Build history of the part. All positions in model axes, mm. A direction names the side the tool comes from. Give positions to 0.01 mm unless a question says otherwise; leave off trailing zeros. Loops run counter-clockwise (first coordinate to the right, second up) from the corner with the lowest first, then second, coordinate; pieces in that order, holes last.
1) Flat gauge pins, fed straight in: P1, Ø2.5, axis at y = 100, z = 2.5, coming from the +X side; P2, Ø3, axis at x = 21, z = 3, coming from the +Y side; P3, Ø1.5, axis at y = -6, z = 2.5, coming from the +X side. Where does each tip first touch, or does it go through?
2) Wall check: line 1 (X direction, y = 82, z = 1.9); line 2 (X direction, y = -49, z = 2.5); line 3 (X direction, y = -6, z = 1.35). Give the ranges that are in metal, low to high.
3) Band-saw the part on A-A on y = -64. List the corners of the cut face in (x, z).
4) Two-plate mould, pull along X, no slides. Class faces 4 (the flat face through (114.786, 13, 2)), 5 (the flat face through (120, -28.788, 2)), 6 (the flat face through (-53.937, -71.013, 2.465)): +X half, -X half, draft (parallel to the pull), parting line (faces both ways), or undercut.
5) Band-saw the part on C-C on x = 64. List the corners of the cut face in (y, z), then the cut area to 3 significant figures.
6) 3-axis set-ups, long thin cutter, end or side, ignore diameter. For faces 1 (the flat face through (120, 56.559, 2)), 2 (the flat face through (-35.311, 68, 3)), 3 (the flat face through (-116.638, 14, 2)): which of +Z, -Z, +X, -X, +Y, -Y reach the whole face in a straight line?
7) Band-saw the part on B-B on y = -10. List the corners of the cut face in (x, z), then the cut area to 3 significant figures.
8) Band-saw the part on D-D on y = 89. List the corners of the cut face in (x, z), then the cut area to 3 significant figures.
```python
from build123d import *

# Parameters (mm, degrees)
BOSS_EXTRUDE1_DEPTH = 5
SKETCH2_W           = 70.400327135
SKETCH2_H           = 34
SKETCH2_R           = 1.6
SKETCH2_R_2         = 4.25
BOSS_EXTRUDE2_DEPTH = 5
SKETCH3_W           = 34.735720487
SKETCH3_H           = 8.029761027
BOSS_EXTRUDE3_DEPTH = 5
BOSS_EXTRUDE4_DEPTH = 5


with BuildPart() as part:
    # Sketch1 → Boss-Extrude1 (new body)
    with BuildSketch(Plane.XY):
        with BuildLine():
            Line((-91.722809189, 104.356193097), (-126.458529676, 104.356193097))
            Line((-126.458529676, 104.356193097), (-126.475267186, 84.614358359))
            Line((-126.475267186, 84.614358359), (-126.480371779, 71.180735955))
            Line((-126.480371779, 71.180735955), (-126.480681684, 56.559478315))
            Line((-126.480681684, 56.559478315), (-116.63815349, 56.559478315))
            Line((-116.63815349, 56.559478315), (-116.63815349, -28.787570067))
            Line((-116.63815349, -28.787570067), (-126.481949379, -28.787570067))
            Line((-126.481949379, -28.787570067), (-126.481949379, -101.34405192))
            Line((-126.481949379, -101.34405192), (-71.448987089, -101.34405192))
            Line((-71.448987089, -101.34405192), (-35.928248301, -39.820327617))
            Line((-35.928248301, -39.820327617), (34.075825089, -39.820327617))
            Line((34.075825089, -39.820327617), (69.596563877, -101.34405192))
            Line((69.596563877, -101.34405192), (124.629526167, -101.34405192))
            Line((124.629526167, -101.34405192), (124.629526167, -28.787570067))
            Line((124.629526167, -28.787570067), (114.912707304, -28.787570067))
            ThreePointArc((114.912707304, -28.787570067), (114.822920988, -28.750379358), (114.785730279, -28.660593042))
            Line((114.785730279, -28.660593042), (114.785730279, 56.432501289))
            ThreePointArc((114.785730279, 56.432501289), (114.822920988, 56.522287605), (114.912707304, 56.559478315))
            Line((114.912707304, 56.559478315), (124.628258473, 56.559478315))
            Line((124.628258473, 56.559478315), (124.627948781, 71.170673702))
            Line((124.627948781, 71.170673702), (124.622835448, 84.62441506))
            Line((124.622835448, 84.62441506), (124.606106464, 104.356193097))
            Line((124.606106464, 104.356193097), (89.870385977, 104.356193097))
            ThreePointArc((89.870385977, 104.356193097), (65.84204117, 79.034177757), (35.089604597, 62.515901216))
            Line((35.089604597, 62.515901216), (35.089604597, 40.385954124))
            Line((35.089604597, 40.385954124), (-35.310722538, 40.385954124))
            Line((-35.310722538, 40.385954124), (-35.310722538, 61.964889462))
            ThreePointArc((-35.310722538, 61.964889462), (-67.008229873, 78.514287134), (-91.722809189, 104.356193097))
        make_face()
    extrude(amount=BOSS_EXTRUDE1_DEPTH)

    # Sketch2 → Boss-Extrude2 (add)
    with BuildSketch(Plane.XY.offset(5)):
        with Locations((-0.11055897, 57.385954124)):
            Rectangle(SKETCH2_W, SKETCH2_H)
        with Locations((-27.3906777, 70.850420218)):
            Circle(SKETCH2_R, mode=Mode.SUBTRACT)
        with Locations((-27.3906777, 49.92148803)):
            Circle(SKETCH2_R, mode=Mode.SUBTRACT)
        with Locations((25.538254488, 49.92148803)):
            Circle(SKETCH2_R, mode=Mode.SUBTRACT)
        with Locations((25.538254488, 70.850420218)):
            Circle(SKETCH2_R, mode=Mode.SUBTRACT)
        with Locations((-13.426211606, 60.385954124)):
            Circle(SKETCH2_R_2, mode=Mode.SUBTRACT)
        with Locations((11.573788394, 60.385954124)):
            Circle(SKETCH2_R_2, mode=Mode.SUBTRACT)
    extrude(amount=-BOSS_EXTRUDE2_DEPTH)

    # Sketch3 → Boss-Extrude3 (add)
    with BuildSketch(Plane.XY.offset(5)):
        with Locations((-109.090669433, 108.371073611)):
            Rectangle(SKETCH3_W, SKETCH3_H)
        with Locations((107.238246221, 108.371073611)):
            Rectangle(SKETCH3_W, SKETCH3_H)
    extrude(amount=-BOSS_EXTRUDE3_DEPTH)

    # Sketch4 → Boss-Extrude4 (add)
    with BuildSketch(Plane.XY.offset(5)):
        with BuildLine():
            Line((89.870385977, 112.385954124), (81.785730279, 112.385954124))
            Line((81.785730279, 112.385954124), (81.785730279, 93.935580042))
            ThreePointArc((81.785730279, 93.935580042), (85.984378147, 99.024608337), (89.870385977, 104.356193097))
            Line((89.870385977, 104.356193097), (89.870385977, 112.385954124))
        make_face()
        with BuildLine():
            Line((-91.722809189, 112.385954124), (-91.722809189, 104.356193097))
            ThreePointArc((-91.722809189, 104.356193097), (-87.836801358, 99.024608337), (-83.63815349, 93.935580042))
            Line((-83.63815349, 93.935580042), (-83.63815349, 112.385954124))
            Line((-83.63815349, 112.385954124), (-91.722809189, 112.385954124))
        make_face()
    extrude(amount=-BOSS_EXTRUDE4_DEPTH)


solid = part.part
```
Findings below:
1. P1: stops at x = 124.61
1. P2: stops at y = 74.39
1. P3: stops at x = 114.79
2. line 1: x = -126.48 to -71.41, 69.56 to 124.62
2. line 2: x = -126.48 to -41.23, 39.38 to 124.63
2. line 3: x = -116.64 to 114.79
3. outline: (-126.48, 0) - (-49.89, 0) - (-49.89, 5) - (-126.48, 5) - close; (48.04, 0) - (124.63, 0) - (124.63, 5) - (48.04, 5) - close
4. face 4: +X half
4. face 5: draft
4. face 6: undercut
5. outline: (-91.65, 0) - (77.66, 0) - (77.66, 5) - (-91.65, 5) - close
5. area: 847 mm2
6. face 1: +Z, -Z, +X
6. face 2: +Z, -Z, +Y
6. face 3: +Z, -Z, -X
7. outline: (-116.64, 0) - (114.79, 0) - (114.79, 5) - (-116.64, 5) - close
7. area: 1,160 mm2
8. outline: (-126.47, 0) - (-79.04, 0) - (-79.04, 5) - (-126.47, 5) - close; (77.18, 0) - (124.62, 0) - (124.62, 5) - (77.18, 5) - close
8. area: 474 mm2
